Source: CAD feature listing. Evaluate the final solid. Frame: model axes, mm. A direction names the side the tool comes from. Give positions to 0.01 mm unless a question says otherwise; leave off trailing zeros. Loops run counter-clockwise (first coordinate to the right, second up) from the corner with the lowest first, then second, coordinate; pieces in that order, holes last. Notation, with made-up numbers: (89, 51.5) -> (137, 51.5) arc R6 ccw to (137, 56.5) -> close; hole circle Ø10 at (2.25, 82.5). An arc over 180 degrees is marked (long way). Return JSON: item names as keys, results as strings. Group by question number.
(1) Cut plane D-D on y = 45. Return loops of the section in (x, z).
(2) Ray query, line 1 (Y direction, x = -57.5, z = -13.5); line 2 (Z direction, x = -97, y = -18); line 3 (X direction, y = -93.5, z = -8). Return the intervals inside material, ascending. Write a range as from..to.
(3) Cut plane B-B on y = -47.5. Return loops of the section in (x, z).
(4) Access query for faces 4 (the face through (-102.431, -26, 1)), 5 (the face through (-97.431, -61, -5)). Directions: +Z, -Z, +X, -X, +Y, -Y. A direction counts if a zero-diameter tool reaches every point of the face in a straight line with its end or side. Return the directions, or none.
(5) Cut plane A-A on x = -68.5. Return loops of the section in (y, z), then the cut area to 3 significant figures.
(6) Cut plane C-C on z = -13.5. Return loops of the section in (x, y), then the cut area to 3 significant figures.
(7) Draft query along Y for faces 1 (the face through (-100, -59, -10)), 2 (the face through (-68, 110, -7)), 3 (the face through (-100, -10, -5)). Return one class per face: released by +Y, released by -Y, zero draft, split by the parting line, or undercut.
(8) Pin query (flat end, axial travel): pin 1 (2 mm diameter, centred on y = -49.5, z = -7, fed in from +X); pin 2 (1 mm diameter, centred on x = -86, z = -1.5, fed in from -Y); pin 3 (4 mm diameter, centred on x = -67, y = -85, fed in from -Z). Return the tip coordinate at first contact, or that it passes through.
```python
from build123d import *

# Parameters (mm, degrees)
SKETCH3_W           = 70
SKETCH3_H           = 220
BOSS_EXTRUDE2_DEPTH = 5
SKETCH4_W           = 5
SKETCH4_H           = 100
BOSS_EXTRUDE3_DEPTH = 10
SKETCH5_W           = 70
SKETCH5_H           = 5
BOSS_EXTRUDE4_DEPTH = 20


with BuildPart() as part:
    # Sketch3 → Boss-Extrude2 (new body)
    with BuildSketch(Plane.XY):
        with Locations((-67.431106164, 0)):
            Rectangle(SKETCH3_W, SKETCH3_H)
    extrude(amount=BOSS_EXTRUDE2_DEPTH)

    # Sketch4 → Boss-Extrude3 (add)
    with BuildSketch(Plane.XY):
        with Locations((-99.931106164, -60)):
            Rectangle(SKETCH4_W, SKETCH4_H)
    extrude(amount=-BOSS_EXTRUDE3_DEPTH)

    # Sketch5 → Boss-Extrude4 (add)
    with BuildSketch(Plane.XY):
        with Locations((-67.431106164, 107.5)):
            Rectangle(SKETCH5_W, SKETCH5_H)
    extrude(amount=-BOSS_EXTRUDE4_DEPTH)


solid = part.part
```
Answers:
{
 "1": {"outline": "(-102.43, 0) -> (-32.43, 0) -> (-32.43, 5) -> (-102.43, 5) -> close"},
 "2": {"line 1": "105..110", "line 2": "0..5", "line 3": "-102.43..-97.43"},
 "3": {"outline": "(-102.43, -10) -> (-97.43, -10) -> (-97.43, 0) -> (-32.43, 0) -> (-32.43, 5) -> (-102.43, 5) -> close"},
 "4": {"face 4": "+Z, -Z, -X, +Y, -Y", "face 5": "-Z, +X, -Y"},
 "5": {"outline": "(-110, 0) -> (105, 0) -> (105, -20) -> (110, -20) -> (110, 5) -> (-110, 5) -> close", "area": "1,200 mm²"},
 "6": {"outline": "(-102.43, 105) -> (-32.43, 105) -> (-32.43, 110) -> (-102.43, 110) -> close", "area": "350 mm²"},
 "7": {"face 1": "zero draft", "face 2": "released by +Y", "face 3": "undercut"},
 "8": {"pin 1": "x = -97.43", "pin 2": "y = 105", "pin 3": "z = 0"}
}
